Input: part model. Units: mm. Frame: model coordinates. A direction names the side the tool comes from. Round coordinates to 2 decimals unless told otherwise and drop trailing zeros. Write each loop counter-clockwise with the first axis right and the second up, starting at its lowest first coordinate (ties: lowest second). Pieces come first, ordered by that corner, then holes. Notation, with made-up numbers: (60, 63.25) - (88, 63.25) arc R34 cw to (88, 100.25) - close; hole circle Ø3 at (38.25, 50.5). An arc over 180 degrees is marked (long way). Use one line per item in the form item = value.
```python
from build123d import *

# Parameters (mm, degrees)
SKETCH013_R      = 1.9
EXTRUDE012_DEPTH = 5
EXTRUDE013_DEPTH = 4


with BuildPart() as extrude012:
    # Sketch013 → Extrude012 (new body)
    with BuildSketch(Plane.XY):
        with BuildLine():
            Line((-37.200665, 15.536565), (-37.258781, -15.414486))
            ThreePointArc((-38.626377, -16.779517), (-37.660247, -16.379864), (-37.258781, -15.414486))
            Line((-38.626377, -16.779517), (-49.200665, -16.779517))
            Line((-49.200665, 16.906731), (-49.200665, -16.779517))
            Line((-38.56826, 16.906731), (-49.200665, 16.906731))
            ThreePointArc((-37.200665, 15.536565), (-37.600315, 16.505263), (-38.56826, 16.906731))
        make_face()
        with Locations((-41, 10)):
            Circle(SKETCH013_R, mode=Mode.SUBTRACT)
        with Locations((-41, -10)):
            Circle(SKETCH013_R, mode=Mode.SUBTRACT)
    extrude(amount=EXTRUDE012_DEPTH)


with BuildPart() as extrude012_1:
    # Extrude012 placement: moved
    add(extrude012.part.moved(Location((0, 0, 11.5))))


with BuildPart() as obj1:
    # Sketch014 (on Face5 of Extrude012) → Extrude013 (new body)
    with BuildSketch(Plane(origin=(-49.200665, 0, 11.5), x_dir=(0, -1, 0), z_dir=(-1, 0, 0))):
        with BuildLine():
            Line((-16.821022, 0), (16.821022, 0))
            Line((16.821022, 0), (16.821022, 15.410553))
            ThreePointArc((16.821022, 15.410553), (16.062591, 17.241569), (14.231576, 18))
            Line((-14.231576, 18), (14.231576, 18))
            ThreePointArc((-14.231576, 18), (-16.062591, 17.241569), (-16.821022, 15.410553))
            Line((-16.821022, 0), (-16.821022, 15.410553))
        make_face()
    extrude(amount=-EXTRUDE013_DEPTH)

    # Fusion013: union Extrude012
    add(extrude012_1.part)


solid = obj1.part
```
(1) Cut plane B-B on y = 10. Output: boundary loops of the cut face in (x, z).
Derived:
outline = (-49.2, 11.5) - (-42.9, 11.5) - (-42.9, 16.5) - (-45.2, 16.5) - (-45.2, 29.5) - (-49.2, 29.5) - close; (-39.1, 11.5) - (-37.21, 11.5) - (-37.21, 16.5) - (-39.1, 16.5) - close
(2) Cut plane D-D on z = 24. Output: boundary loops of the cut face in (x, y), then the cut area to 3 significant figures.
Derived:
outline = (-49.2, -16.82) - (-45.2, -16.82) - (-45.2, 16.82) - (-49.2, 16.82) - close
area = 135 mm^2
(3) Draft query along X for faces 1 (the face through (-47.2, 16, 28.8)), 2 (the face through (-39.245, 9.272, 13.965)), 3 (the face through (-39.245, -10.728, 13.965)), 4 (the face through (-37.59, 16.495, 13.965)). Return one class per face: released by +X, released by -X, zero draft, split by the parting line, or undercut.
Derived:
face_1 = zero draft
face_2 = undercut
face_3 = undercut
face_4 = released by +X
(4) Material intervals for L1, parallel to Y at x = -41, z = 13.3; L2, parallel to X at y = 9, z = 21.5; L3, parallel to Z at x = -41.25, y = 0, sorted ascending.
Derived:
L1 = -16.78 to -11.9, -8.1 to 8.1, 11.9 to 16.91
L2 = -49.2 to -45.2
L3 = 11.5 to 16.5
(5) Cut plane A-A on x = -41. Output: boundary loops of the cut face in (y, z), then the cut area to 3 significant figures.
Derived:
outline = (-16.78, 11.5) - (-11.9, 11.5) - (-11.9, 16.5) - (-16.78, 16.5) - close; (-8.1, 11.5) - (8.1, 11.5) - (8.1, 16.5) - (-8.1, 16.5) - close; (11.9, 11.5) - (16.91, 11.5) - (16.91, 16.5) - (11.9, 16.5) - close
area = 130 mm^2
(6) Access query for faces 5 (the face through (-47, 16.821, 22)), 6 (the face through (-42, -16.78, 14)), 7 (the face through (-43, 0, 11.5)). Directions: +Z, -Z, +X, -X, +Y, -Y. A direction counts if a zero-diameter tool reaches every point of the face in a straight line with its end or side. Return the directions, or none.
Derived:
face_5 = +Z, +X, -X, +Y
face_6 = +Z, -Z, +X, -Y
face_7 = -Z, +X, -X, +Y, -Y
(7) Cut plane C-C on y = -11.5. Output: boundary loops of the cut face in (x, z), then the cut area to 3 significant figures.
Derived:
outline = (-49.2, 11.5) - (-42.17, 11.5) - (-42.17, 16.5) - (-45.2, 16.5) - (-45.2, 29.5) - (-49.2, 29.5) - close; (-39.83, 11.5) - (-37.25, 11.5) - (-37.25, 16.5) - (-39.83, 16.5) - close
area = 100 mm^2
(8) First-contact query: pin 1 Ø2 at (x, z) = (-48, 22) entering from +Y; pin 2 Ø4 at (y, z) = (-12, 27) entering from +X; pin 3 Ø5.5 at (x, z) = (-42, 13) entering from -Y. Flat tips, straight axial feed; report the tip coordinate or a pass-through.
Derived:
pin_1 = 16.82
pin_2 = -45.2
pin_3 = -16.78
